Autodesk Inventor part; units mm, degrees
ref_plane "YZ Plane" through (0, 0, 0) normal (1, 0, 0) x (0, 1, 0)
ref_plane "XZ Plane" through (0, 0, 0) normal (0, 1, 0) x (-1, 0, 0)
ref_plane "XY Plane" through (0, 0, 0) normal (0, 0, 1) x (1, 0, 0)
ref_plane "РабПлоскость2" through (-682.985, -17.9529, 102.0837) normal (0, 1, 0) x (-1, 0, 0)
ref_plane "РабПлоскость3" through (1272.2614, -51.4529, 81.5837) normal (0, 0, 1) x (1, 0, 0)
sketch "Эскиз1" plane through (1272.2614, -51.4529, 81.5837) normal (0, 0, 1) x (1, 0, 0)
  point P0 (-1272.2614, 51.4529)
sketch "Эскиз2" plane through (-682.985, -17.9529, 102.0837) normal (0, 1, 0) x (-1, 0, 0)
  line L0 (-11.5, -11.5) -> (11.5, -11.5)
  line L1 (11.5, -11.5) -> (11.5, 11.5)
  line L2 (11.5, 11.5) -> (-11.5, 11.5)
  line L3 (-11.5, 11.5) -> (-11.5, -11.5)
  line L4 (-11.5, -11.5) -> (11.5, 11.5) construction
  line L5 (11.5, -11.5) -> (-11.5, 11.5) construction
  circle A0 centre (8.5, 8.5) radius 2
  circle A1 centre (8.5, -8.5) radius 2
  line L6 (0, 20.5912) -> (0, -22.1181)
  circle A2 centre (-8.5, 8.5) radius 2
  circle A3 centre (-8.5, -8.5) radius 2
  point P0 (-682.985, -102.0837)
  point P1 (0, 0)
  point P2 (0, 0)
  dimension "d0" = 23
  dimension "d1" = 23
  dimension "d2" = 4
  dimension "d5" = 3
  dimension "d6" = 3
  dimension "d7" = 4
  dimension "d8" = 3
  dimension "d9" = 3
extrude "Выдавливание1" add sketch "Эскиз2" along normal blind 2
sketch "Эскиз3" plane through (-694.485, -17.9529, 90.5837) normal (-1, 0, 0) x (0, 0, 1)
  line L0 (23, 0) -> (0, 0)
  line L1 (23, 2) -> (0, 2)
  line L2 (0, 2) -> (0, 0)
  line L3 (0, 0) -> (23, 0)
  line L4 (23, 0) -> (23, 2)
  point P0 (-90.5837, 17.9529)
extrude "Выдавливание2" add sketch "Эскиз3" along normal blind 12
sketch "Эскиз6" plane through (-706.485, -17.9529, 90.5837) normal (-1, 0, 0) x (0, 0, 1)
  line L0 (23, 2) -> (0, 2)
  line L1 (0, 2) -> (0, -31.5)
  line L2 (0, -31.5) -> (23, -31.5)
  line L3 (23, -31.5) -> (23, 2)
  point P0 (-90.5837, 17.9529)
  dimension "d14" = 33.5
extrude "Выдавливание3" add sketch "Эскиз6" along normal blind 2
sketch "Эскиз7" plane through (-671.485, -17.9529, 113.5837) normal (1, 0, 0) x (0, 0, -1)
  point P0 (113.5837, 17.9529)
sketch "Эскиз8" plane through (-682.985, -17.9529, 102.0837) normal (0, 1, 0) x (-1, 0, 0)
  point P0 (-682.985, -102.0837)
sketch "Эскиз9" plane through (-671.485, -17.9529, 113.5837) normal (1, 0, 0) x (0, 0, -1)
  line L0 (23, 0) -> (23, 2)
  line L1 (23, 2) -> (0, 2)
  line L2 (0, 2) -> (0, 0)
  line L3 (0, 0) -> (23, 0)
  line L4 (23, 0) -> (23, 2)
  point P0 (113.5837, 17.9529)
extrude "Выдавливание4" add sketch "Эскиз9" along normal blind 12
sketch "Эскиз10" plane through (-659.485, -17.9529, 113.5837) normal (1, 0, 0) x (0, 0, -1)
  line L0 (0, 2) -> (23, 2)
  line L1 (23, -31.5) -> (0, -31.5)
  line L2 (23, 2) -> (0, 2)
  line L3 (0, 2) -> (0, -31.5)
  line L4 (0, -31.5) -> (23, -31.5)
  line L5 (23, -31.5) -> (23, 2)
  point P0 (113.5837, 17.9529)
  point P1 (23, -31.5)
extrude "Выдавливание5" add sketch "Эскиз10" along normal blind 2
sketch "Эскиз11" plane through (-682.985, -15.9529, 102.0837) normal (0, 1, 0) x (1, 0, 0)
  line L0 (6.5, -6.5) -> (-6.5, -6.5)
  line L1 (-6.5, -6.5) -> (-6.5, 6.5)
  line L2 (-6.5, 6.5) -> (6.5, 6.5)
  line L3 (6.5, 6.5) -> (6.5, -6.5)
  line L4 (6.5, -6.5) -> (-6.5, 6.5) construction
  line L5 (-6.5, -6.5) -> (6.5, 6.5) construction
  point P0 (682.985, 102.0837)
  point P1 (0, 0)
  point P2 (0, 0)
  dimension "d21" = 13
  dimension "d22" = 13
extrude "Выдавливание6" cut sketch "Эскиз11" against normal blind 10
ref_plane "РабПлоскость4" through (-602.7943, -49.4529, 186.5837) normal (0, 1, 0) x (-1, 0, 0)
sketch "Эскиз12" plane through (-602.7943, -49.4529, 186.5837) normal (0, 1, 0) x (-1, 0, 0)
  circle A0 centre (114.5237, -85) radius 2
  circle A1 centre (62.5237, -85) radius 2
  line L0 (56.6907, -73) -> (56.6907, -96)
  line L1 (56.6907, -73) -> (121.6907, -73)
  line L2 (121.6907, -73) -> (121.6907, -96)
  line L3 (121.6907, -96) -> (56.6907, -96)
  line L4 (56.6907, -96) -> (56.6907, -73)
  line L5 (105.6907, -73) -> (105.6907, -96)
  point P0 (-602.7943, -186.5837)
  dimension "d25" = 65
extrude "Выдавливание8" add sketch "Эскиз12" along normal blind 2 contours L1 L2 L3 L5
ref_plane "РабПлоскость5" through (-602.7943, -49.4529, 186.5837) normal (0, 1, 0) x (-1, 0, 0)
sketch "Эскиз13" plane through (-602.7943, -49.4529, 186.5837) normal (0, 1, 0) x (-1, 0, 0)
  line L0 (54.6907, -96) -> (54.6907, -73)
  line L1 (54.6907, -73) -> (41.9796, -73)
  line L2 (41.9796, -73) -> (41.9796, -96)
  line L3 (41.9796, -96) -> (54.6907, -96)
  line L4 (54.6907, -96) -> (54.6907, -73)
  circle A0 centre (52.55, -84.25) radius 1
  point P0 (-602.7943, -186.5837)
extrude "Выдавливание9" add sketch "Эскиз13" along normal blind 2
sketch "Эскиз14" plane through (-682.985, -15.9529, 102.0837) normal (0, 1, 0) x (1, 0, 0)
  line L0 (10, -10) -> (-10, -10)
  line L1 (-10, -10) -> (-10, 10)
  line L2 (-10, 10) -> (10, 10)
  line L3 (10, 10) -> (10, -10)
  line L4 (10, -10) -> (-10, 10) construction
  line L5 (-10, -10) -> (10, 10) construction
  point P0 (682.985, 102.0837)
  point P1 (0, 0)
  point P2 (0, 0)
  dimension "d32" = 20
  dimension "d33" = 20
extrude "Выдавливание10" cut sketch "Эскиз14" against normal blind 10
properties part number "деталь крепление энкодера"
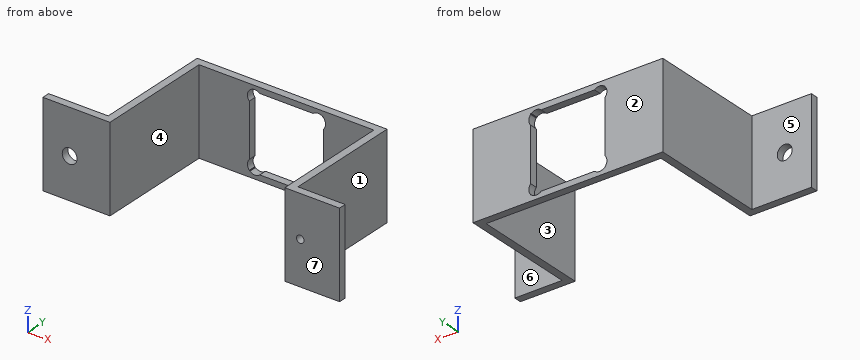
Input: part model. Units: mm. Frame: model coordinates. Face numbers are marked on the shaded views. A direction names the side the tool comes from. Give positions to 0.01 mm unless a question says otherwise; leave off trailing zeros. Write each loop counter-clockwise with the first axis right and the second up, starting at its lowest first coordinate (ties: lowest second). Pieces come first, ordered by that corner, then holes. Notation, with made-up numbers: (64, 41.5) -> (109, 41.5) arc R21 ccw to (109, 76.5) -> close; hole circle Ø9 at (-16.5, 24). An arc over 180 degrees is marked (long way). Use one line per item in the form item = value. Start each with the question number.
1) Set-up query: the marked faces 4, 5, 6 and 7. Return all of +Z, -Z, +X, -X, +Y, -Y with unobstructed straight access to the full face (end or side cutting, diameter ignored); none if empty.
2) Section query B-B on x = -684.5. Return the cut outline in (y, z), then the cut area to 3 significant figures.
3) Section query D-D on x = -650. Return the cut outline in (y, z).
4) Draft query along X for the marked faces 1, 2 and 3. Return one class per face: pulls with the +X half, pulls with the -X half, needs draft (parallel to the pull), parting line crosses it, or undercut.
5) Section query C-C on z = 98. Return the cut outline in (x, y) (3 decimals).
6) Ray query, probe 1 along X at (y, z) = (-27, 99.5) (3 decimals); probe 2 along Y at (x, z) = (-649, 112.25); probe 3 along Y at (x, z) = (-668, 101). Return the intervals inside material, ascending. Write a range as from..to.
7) Section query A-A on y = -44. Return the cut outline in (x, z) (3 decimals).
8) Pin query (flat end, axial travel): pin 1 (5 mm diameter, centred on y = -29.5, z = 100.5, fed in from -X) (3 decimals); pin 2 (2 mm diameter, centred on x = -715.5, z = 97.5, fed in from +Y); pin 3 (8 mm diameter, centred on x = -694, z = 101.5, fed in from -Y). Return the tip coordinate at first contact, or that it passes through.
Outcome:
q1.face_4 = +Z, -Z, -Y
q1.face_5 = +Z, -Z, -X, +Y
q1.face_6 = +Z, -Z, +X, +Y
q1.face_7 = +Z, -Z, +X, -X, -Y
q2.outline = (-17.95, 90.58) -> (-15.95, 90.58) -> (-15.95, 92.08) -> (-17.95, 92.08) -> close; (-17.95, 112.08) -> (-15.95, 112.08) -> (-15.95, 113.58) -> (-17.95, 113.58) -> close
q2.area = 6.00 mm^2
q3.outline = (-49.45, 90.58) -> (-47.45, 90.58) -> (-47.45, 113.58) -> (-49.45, 113.58) -> close
q4.face_1 = pulls with the +X half
q4.face_2 = needs draft
q4.face_3 = undercut
q5.outline = (-724.485, -49.453) -> (-706.485, -49.453) -> (-706.485, -17.953) -> (-692.985, -17.953) -> (-692.985, -15.953) -> (-708.485, -15.953) -> (-708.485, -47.453) -> (-724.485, -47.453) -> close; (-672.985, -17.953) -> (-659.485, -17.953) -> (-659.485, -49.453) -> (-644.774, -49.453) -> (-644.774, -47.453) -> (-657.485, -47.453) -> (-657.485, -15.953) -> (-672.985, -15.953) -> close
q6.probe_1 = -708.485..-706.485, -659.485..-657.485
q6.probe_2 = -49.45..-47.45
q6.probe_3 = -17.95..-15.95
q7.outline = (-708.485, 90.584) -> (-706.485, 90.584) -> (-706.485, 113.584) -> (-708.485, 113.584) -> close; (-659.485, 90.584) -> (-657.485, 90.584) -> (-657.485, 113.584) -> (-659.485, 113.584) -> close
q8.pin_1 = -708.485
q8.pin_2 = -47.45
q8.pin_3 = -17.95
